The listing builds one solid part. Answer for the finished solid, in the listing's coordinates (mm). Face numbers are marked on the shaded views. A direction names the side the tool comes from. Round coordinates to 2 decimals unless told otherwise and drop trailing zeros. Write each loop counter-clockwise with the first axis right and the second up, starting at its lowest first coordinate (ties: lowest second). Pieces come first, ordered by that corner, then holes.
(1) A cutting plane is placed at C-C, the plane y = -22.8. Give the vertices of the cut face in (x, z), and give its area (3 significant figures).
(2) A cutting plane is placed at B-B, the plane z = 18. Give the vertices of the cut face in (x, y), and give its area (3 significant figures).
(3) Each of these flat-tipped pins is pushed along its axis until it touches: pin 1 Ø6 at (x, y) = (5.5, -3.5) entering from +Z; pin 2 Ø1.6 at (x, z) = (4, 25) entering from -Y; pin 3 Ø1 at (x, z) = (3.5, -5.5) entering from -Y; pin 4 Ø2.5 at (x, z) = (5, -16) entering from -Y. Where does it stop, or does it pass through?
(4) A cutting plane is placed at A-A, the plane y = -16.75. Give the vertices of the cut face in (x, z).
(5) A cutting plane is placed at D-D, the plane x = 13. Give the vertices of the cut face in (y, z).
(6) Find the intervals of material crossed by probe 1 along Z at (x, y) = (7, -8.05); probe 2 along Z at (x, y) = (10, -13); probe 3 along Z at (x, y) = (7, -3.8), in increasing order.
(7) The mould has two halves that part along Z. Classify the marked faces 1, 2, 3 and 4: +Z half, -Z half, draft (parallel to the pull), parting line (faces both ways), or undercut.
(8) For the marked faces 5, 6 and 7, determine the directions among +Z, -Z, +X, -X, +Y, -Y from which every point of the face is accessible in a straight line to the end or side of a thin tool.
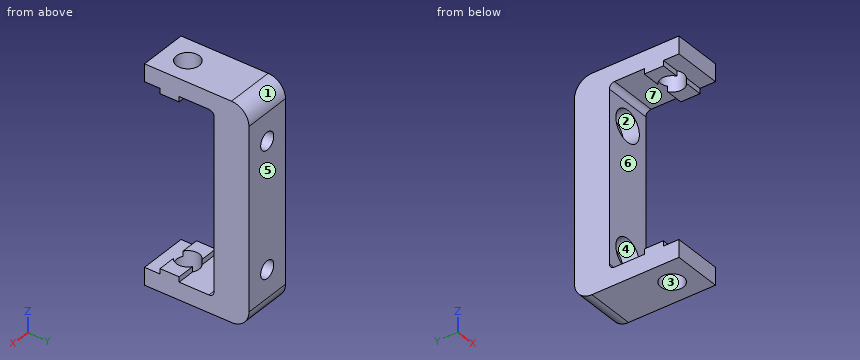
from build123d import *

# Parameters (mm, degrees)
BOSS_EXTRUDE1_DEPTH  = 14
SKETCH4_W            = 14
SKETCH4_H            = 5.5
BOSS_EXTRUDE3_DEPTH  = 1.5
CUT_EXTRUDE1_START   = -6.5
SKETCH2_R            = 3.3
CUT_EXTRUDE1_DEPTH   = 6.5
FILLET1_R            = 5
FILLET2_R            = 1.5
SKETCH7_R            = 2.5
CUT_EXTRUDE4_DEPTH   = 11
SKETCH7_3_R          = 4.5
SKETCH7_3_R_2        = 2.5
CUT_EXTRUDE5_DEPTH   = 4.6
FILLET1_OF_MIRROR1_R = 5
FILLET2_OF_MIRROR1_R = 1.5


with BuildPart() as part:
    # Sketch1 → Boss-Extrude1 (new body)
    with BuildSketch(Plane(origin=(0, 0, 0), x_dir=(0, 0, -1), z_dir=(1, 0, 0))):
        Polygon((0, 0), (-31, 0), (-31, -30), (-26, -30), (-26, -10), (0, -10), align=None)
    boss_extrude1 = extrude(amount=BOSS_EXTRUDE1_DEPTH)

    # Sketch4 → Boss-Extrude3 (add)
    with BuildSketch(Plane(origin=(0, 0, 26), x_dir=(-1, 0, 0), z_dir=(0, 0, -1))):
        with Locations((-7, -22.8)):
            Rectangle(SKETCH4_W, SKETCH4_H)
    boss_extrude3 = extrude(amount=BOSS_EXTRUDE3_DEPTH)

    # Sketch2 → Cut-Extrude1 (cut)
    with BuildSketch(Plane.XY.offset(31).offset(CUT_EXTRUDE1_START)):
        with Locations((7, -22.8)):
            Circle(SKETCH2_R)
    cut_extrude1 = extrude(amount=CUT_EXTRUDE1_DEPTH, mode=Mode.SUBTRACT)

    # Fillet1
    fillet1_edges = [part.edges().sort_by_distance(p)[0] for p in [
        (7, 0, 31),
    ]]
    fillet(fillet1_edges, radius=FILLET1_R)

    # Fillet2
    fillet2_edges = [part.edges().sort_by_distance(p)[0] for p in [
        (7, -10, 26),
    ]]
    fillet(fillet2_edges, radius=FILLET2_R)

    # Sketch7 → Cut-Extrude4 (cut, through all)
    with BuildSketch(Plane(origin=(0, -10, 0), x_dir=(1, 0, 0), z_dir=(0, 1, 0))):
        with Locations((7, -18)):
            Circle(SKETCH7_R)
    cut_extrude4 = extrude(amount=CUT_EXTRUDE4_DEPTH, mode=Mode.SUBTRACT)

    # Sketch7<3> → Cut-Extrude5 (cut)
    with BuildSketch(Plane(origin=(0, -10, 0), x_dir=(1, 0, 0), z_dir=(0, 1, 0))):
        with Locations((7, -18)):
            Circle(SKETCH7_3_R)
        with Locations((7, -18)):
            Circle(SKETCH7_3_R_2, mode=Mode.SUBTRACT)
    cut_extrude5 = extrude(amount=CUT_EXTRUDE5_DEPTH, mode=Mode.SUBTRACT)

    # Mirror1: Boss-Extrude1, Boss-Extrude3, Cut-Extrude1, Cut-Extrude4, Cut-Extrude5 across plane
    add(boss_extrude1.mirror(Plane.XY))
    add(boss_extrude3.mirror(Plane.XY))
    add(cut_extrude1.mirror(Plane.XY), mode=Mode.SUBTRACT)
    add(cut_extrude4.mirror(Plane.XY), mode=Mode.SUBTRACT)
    add(cut_extrude5.mirror(Plane.XY), mode=Mode.SUBTRACT)

    # Fillet1 of Mirror1
    fillet1_of_mirror1_edges = [part.edges().sort_by_distance(p)[0] for p in [
        (7, 0, -31),
    ]]
    fillet(fillet1_of_mirror1_edges, radius=FILLET1_OF_MIRROR1_R)

    # Fillet2 of Mirror1
    fillet2_of_mirror1_edges = [part.edges().sort_by_distance(p)[0] for p in [
        (7, -10, -26),
    ]]
    fillet(fillet2_of_mirror1_edges, radius=FILLET2_OF_MIRROR1_R)


solid = part.part
Solutions:
1. outline: (0, -31) - (3.7, -31) - (3.7, -24.5) - (0, -24.5) - close; (0, 24.5) - (3.7, 24.5) - (3.7, 31) - (0, 31) - close; (10.3, -31) - (14, -31) - (14, -24.5) - (10.3, -24.5) - close; (10.3, 24.5) - (14, 24.5) - (14, 31) - (10.3, 31) - close
1. area: 96.2 mm2
2. outline: (0, -10) - (2.5, -10) - (2.5, -5.4) - (4.5, -5.4) - (4.5, 0) - (0, 0) - close; (9.5, -5.4) - (11.5, -5.4) - (11.5, -10) - (14, -10) - (14, 0) - (9.5, 0) - close
2. area: 71.6 mm2
3. pin 1: stops at z = 31
3. pin 2: stops at y = -25.55
3. pin 3: stops at y = -10
3. pin 4: stops at y = -5.4
4. outline: (0, -31) - (14, -31) - (14, -26) - (0, -26) - close; (0, 26) - (14, 26) - (14, 31) - (0, 31) - close
5. outline: (-30, -31) - (-5, -31) arc R5 ccw to (0, -26) - (0, 26) arc R5 ccw to (-5, 31) - (-30, 31) - (-30, 26) - (-25.55, 26) - (-25.55, 24.5) - (-20.05, 24.5) - (-20.05, 26) - (-11.5, 26) arc R1.5 cw to (-10, 24.5) - (-10, -24.5) arc R1.5 cw to (-11.5, -26) - (-20.05, -26) - (-20.05, -24.5) - (-25.55, -24.5) - (-25.55, -26) - (-30, -26) - close
6. probe 1: z = -31 to -22.5, -13.5 to 13.5, 22.5 to 31
6. probe 2: z = -31 to -26, 26 to 31
6. probe 3: z = -30.85 to -20.5, -15.5 to 15.5, 20.5 to 30.85
7. face 1: +Z half
7. face 2: undercut
7. face 3: draft
7. face 4: undercut
8. face 5: +Z, -Z, +X, -X, +Y
8. face 6: +X, -X, -Y
8. face 7: +X, -X
